from build123d import *

# Parameters (mm, degrees)
CROQUIS1_R              = 20.5
CROQUIS1_R_2            = 1.5
SALIENTE_EXTRUIR1_DEPTH = 2
CROQUIS2_R              = 11.5
CROQUIS2_R_2            = 9.5
SALIENTE_EXTRUIR2_DEPTH = 8
CROQUIS3_R              = 1.5
CROQUIS3_R_2            = 9.5
SALIENTE_EXTRUIR4_DEPTH = 8
REDONDEO1_R             = 1
CORTAR_EXTRUIR1_DEPTH   = 8


with BuildPart() as part:
    # Croquis1 → Saliente-Extruir1 (new body)
    with BuildSketch(Plane.XY):
        Circle(CROQUIS1_R)
        with Locations((15, 8.1)):
            Circle(CROQUIS1_R_2, mode=Mode.SUBTRACT)
        with Locations((0, -16)):
            Circle(CROQUIS1_R_2, mode=Mode.SUBTRACT)
        with Locations(Location((-15, 8.1, 0), (0, 0, 180))):
            Circle(CROQUIS1_R_2, mode=Mode.SUBTRACT)
    extrude(amount=SALIENTE_EXTRUIR1_DEPTH)

    # Croquis2 → Saliente-Extruir2 (add)
    with BuildSketch(Plane.XY.offset(2)):
        Circle(CROQUIS2_R)
        Circle(CROQUIS2_R_2, mode=Mode.SUBTRACT)
    extrude(amount=SALIENTE_EXTRUIR2_DEPTH)

    # Croquis3 → Saliente-Extruir4 (add)
    with BuildSketch(Plane.XY.offset(2)):
        with BuildLine():
            Line((-15, -11.6), (15, -11.6))
            ThreePointArc((15, -11.6), (18.059663437, -9.799546895), (17.971452283, -6.250548371))
            Line((17.971452283, -6.250548371), (2.971452283, 17.849451629))
            ThreePointArc((2.971452283, 17.849451629), (0, 19.5), (-2.971452283, 17.849451629))
            Line((-2.971452283, 17.849451629), (-17.971452283, -6.250548371))
            ThreePointArc((-17.971452283, -6.250548371), (-18.059663437, -9.799546895), (-15, -11.6))
        make_face()
        with Locations((15, -8.1)):
            Circle(CROQUIS3_R, mode=Mode.SUBTRACT)
        with Locations((-15, -8.1)):
            Circle(CROQUIS3_R, mode=Mode.SUBTRACT)
        with Locations((0, 16)):
            Circle(CROQUIS3_R, mode=Mode.SUBTRACT)
        Circle(CROQUIS3_R_2, mode=Mode.SUBTRACT)
    extrude(amount=SALIENTE_EXTRUIR4_DEPTH)

    # Redondeo1
    redondeo1_edges = [part.edges().sort_by_distance(p)[0] for p in [
        (-10.471452283, 5.799451629, 10),
        (-18.059663437, -9.799546895, 10),
        (0, -11.6, 10),
        (18.059663437, -9.799546895, 10),
        (10.471452283, 5.799451629, 10),
        (0, 19.5, 10),
    ]]
    fillet(redondeo1_edges, radius=REDONDEO1_R)

    # Croquis4 → Cortar-Extruir1 (cut)
    with BuildSketch(Plane.XY.offset(10)):
        with BuildLine():
            Line((-10.236239063, -2.338676942), (-13.199718145, -7.1))
            Line((-13.199718145, -7.1), (-7.735631842, -7.1))
            ThreePointArc((-7.735631842, -7.1), (-9.295944561, -4.882152673), (-10.236239063, -2.338676942))
        make_face()
        with BuildLine():
            Line((2.421529631, 10.216956212), (0, 14.107547153))
            Line((0, 14.107547153), (-2.421529631, 10.216956212))
            ThreePointArc((-2.421529631, 10.216956212), (0, 10.5), (2.421529631, 10.216956212))
        make_face()
        with BuildLine():
            Line((7.735631842, -7.1), (13.199718145, -7.1))
            Line((13.199718145, -7.1), (10.236239063, -2.338676942))
            ThreePointArc((10.236239063, -2.338676942), (9.295944561, -4.882152673), (7.735631842, -7.1))
        make_face()
    extrude(amount=-CORTAR_EXTRUIR1_DEPTH, mode=Mode.SUBTRACT)


solid = part.part
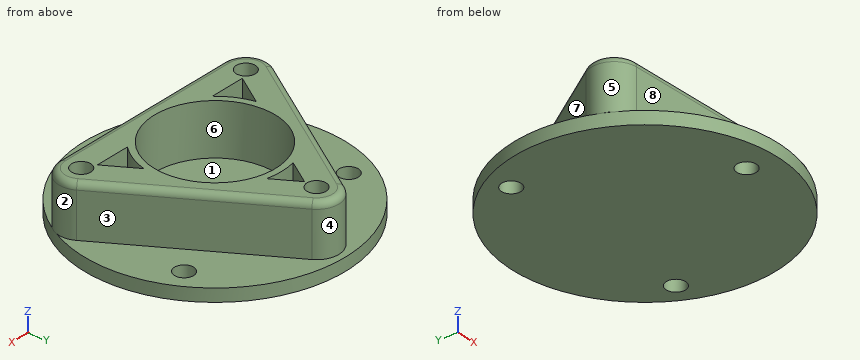
Source: CAD feature listing. Evaluate the final solid. Frame: model axes, mm. Face numbers are marked on the shaded views. A direction names the side the tool comes from. Round coordinates to 2 decimals unless told otherwise and drop trailing zeros. Loops run counter-clockwise (first coordinate to the right, second up) from the corner with the lowest first, then second, coordinate; pieces in that order, holes last. Notation, with made-up numbers: (-35.5, 66.5) - (-12.5, 66.5) arc R22 cw to (-12.5, 103.5) - close; hole circle Ø5 at (27.5, 65). An arc over 180 degrees is marked (long way). Write item = value, one per line. Start each with the question number.
(1) Pin query (flat end, axial travel): pin 1 (4 mm diameter, centred on x = 15, y = 8.1, fed in from +Z); pin 2 (4.5 mm diameter, centred on x = 0, y = 12, fed in from +Z); pin 3 (6 mm diameter, centred on y = -15, z = 6, fed in from +X); pin 4 (3.5 mm diameter, centred on x = 2, z = 5, fed in from -Y). Return the tip coordinate at first contact, or that it passes through.
(2) Section query A-A, the plane z = 7.75. Output: boundary loops of the cut face in (x, y), plus the area to 3 significant figures.
(3) Set-up query: the marked faces 4, 5, 6, 7 and 8. Return all of +Z, -Z, +X, -X, +Y, -Y with unobstructed straight access to the full face (end or side cutting, diameter ignored); none if empty.
(4) Ray query, line 1 along X through (y, z) = (-4, 3); line 2 along X through (y, z) = (-6.5, 5.5); line 3 along Z through (x, y) = (-17.5, -2). Return the intervals inside material, ascending. Write a range as from..to.
(5) Pull-direction query (Y, two-part tool) for the marked faces 1, 2 and 3; classes: +Y half, -Y half, draft (parallel to the pull), parting line (faces both ways), or undercut.
Conclusion:
q1.pin_1 = 2
q1.pin_2 = 10
q1.pin_3 = through
q1.pin_4 = -11.6
q2.outline = (-17.97, -6.25) arc R3.5 ccw to (-15, -11.6) - (15, -11.6) arc R3.5 ccw to (17.97, -6.25) - (2.97, 17.85) arc R3.5 ccw to (-2.97, 17.85) - close; hole circle Ø3 at (-15, -8.1); hole (-13.2, -7.1) - (-7.74, -7.1) arc R10.5 cw to (-10.24, -2.34) - close; hole circle Ø19 at (0, 0); hole (-2.42, 10.22) arc R10.5 cw to (2.42, 10.22) - (0, 14.11) - close; hole circle Ø3 at (0, 16); hole (7.74, -7.1) - (13.2, -7.1) - (10.24, -2.34) arc R10.5 cw to start; hole circle Ø3 at (15, -8.1)
q2.area = 367 mm2
q3.face_4 = +Z, +Y
q3.face_5 = +Z, -X
q3.face_6 = +Z
q3.face_7 = +Z, -X, +Y
q3.face_8 = +Z, +X, -X, -Y
q4.line_1 = -16.57..-11.27, -9.71..-8.62, 8.62..9.71, 11.27..16.57
q4.line_2 = -18.11..-12.83, -8.25..-6.93, 6.93..8.25, 12.83..18.11
q4.line_3 = 0..2
q5.face_1 = undercut
q5.face_2 = parting line
q5.face_3 = +Y half
